For this review, use the dimensioned drawing (mm, ordinates from the lowest corner) and the shaded views. Coordinates: 2 decimals unless noted, no trailing zeros. Loops run counter-clockwise (first coordinate to the right, second up) from the corner with the lowest first, then second, coordinate; pieces in that order, holes last. Notation, with made-up numbers: M 33,-1.75 L 66,-1.75 A13 cw 66,3.25 Z; hole C -3,61.5 d11. An arc over 180 degrees is marked long. One line per item, written item: value.
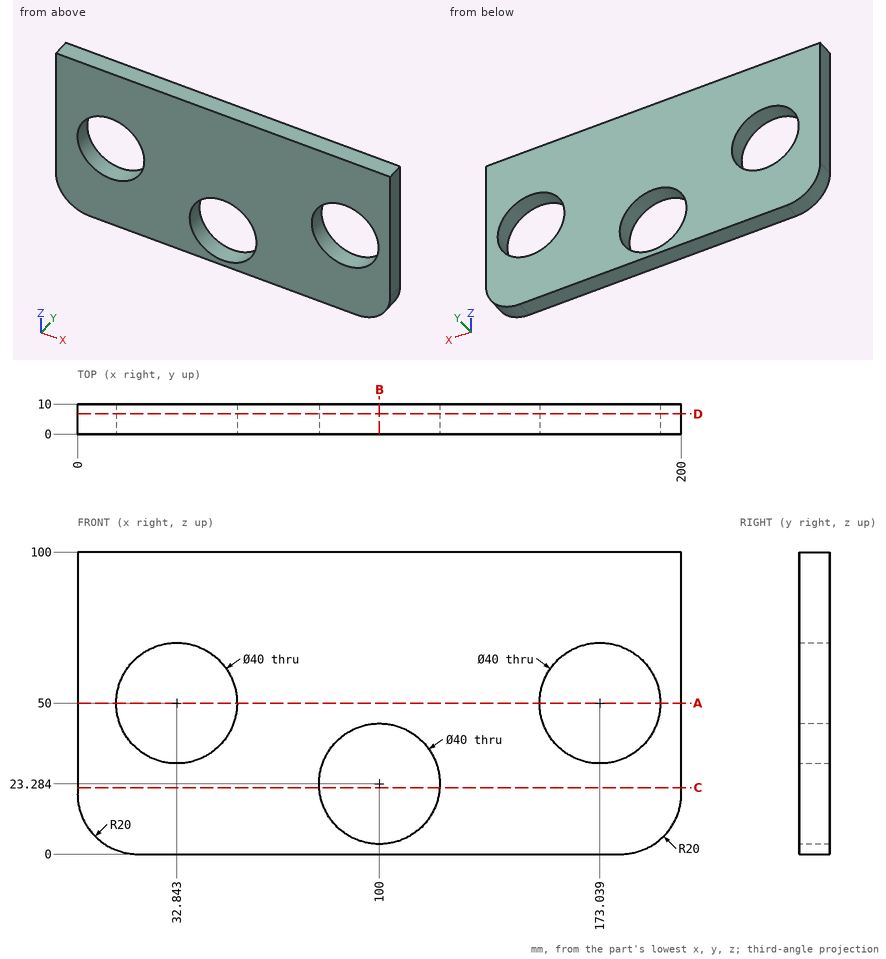
(1) Add section B-B on x = 100. State the section outline as (y, z) points, then the cut area to 3 significant figures.
Checks:
outline: M 0,0 L 10,0 L 10,3.28 L 0,3.28 Z; M 0,43.28 L 10,43.28 L 10,100 L 0,100 Z
area: 600 mm^2
(2) To check wall thickness, follow L1, parallel to X at y = 6.25, z = 50; L2, parallel to X at y = 6.25, z = 45 (1 decimal); L3, parallel to X at y = 9.75, z = 36 (1 decimal). State the ranges of each line that lie inside material, in increasing order. Write a range as [from, to].
Checks:
L1: [0, 12.84], [52.84, 153.04], [193.04, 200]
L2: [0, 13.5], [52.2, 153.7], [192.4, 200]
L3: [0, 18.6], [47.1, 84.6], [115.4, 158.8], [187.3, 200]
(3) Add section A-A on z = 50. State the section outline as (x, y) points.
Checks:
outline: M 0,0 L 12.84,0 L 12.84,10 L 0,10 Z; M 52.84,0 L 153.04,0 L 153.04,10 L 52.84,10 Z; M 193.04,0 L 200,0 L 200,10 L 193.04,10 Z
(4) Add section C-C on z = 22. State the section outline as (x, y) points, then the cut area to 3 significant figures.
Checks:
outline: M 0,0 L 80.04,0 L 80.04,10 L 0,10 Z; M 119.96,0 L 200,0 L 200,10 L 119.96,10 Z
area: 1,600 mm^2
(5) Insertion check: pin 1 Ø1 at (x, z) = (158, 82.5) entering from -Y; pin 2 Ø6 at (y, z) = (5, 15.5) entering from -X. Each pin has a flat end and moves straight along its axis. Give the tip position at first contact, or say it passes through.
Checks:
pin 1: y = 0
pin 2: x = 0.06
(6) Add section D-D on y = 6.75. State the section outline as (x, z) points, then the cut area to 3 significant figures.
Checks:
outline: M 0,20 A20 ccw 20,0 L 180,0 A20 ccw 200,20 L 200,100 L 0,100 Z; hole C 32.84,50 d40; hole C 100,23.28 d40; hole C 173.04,50 d40
area: 16,100 mm^2
